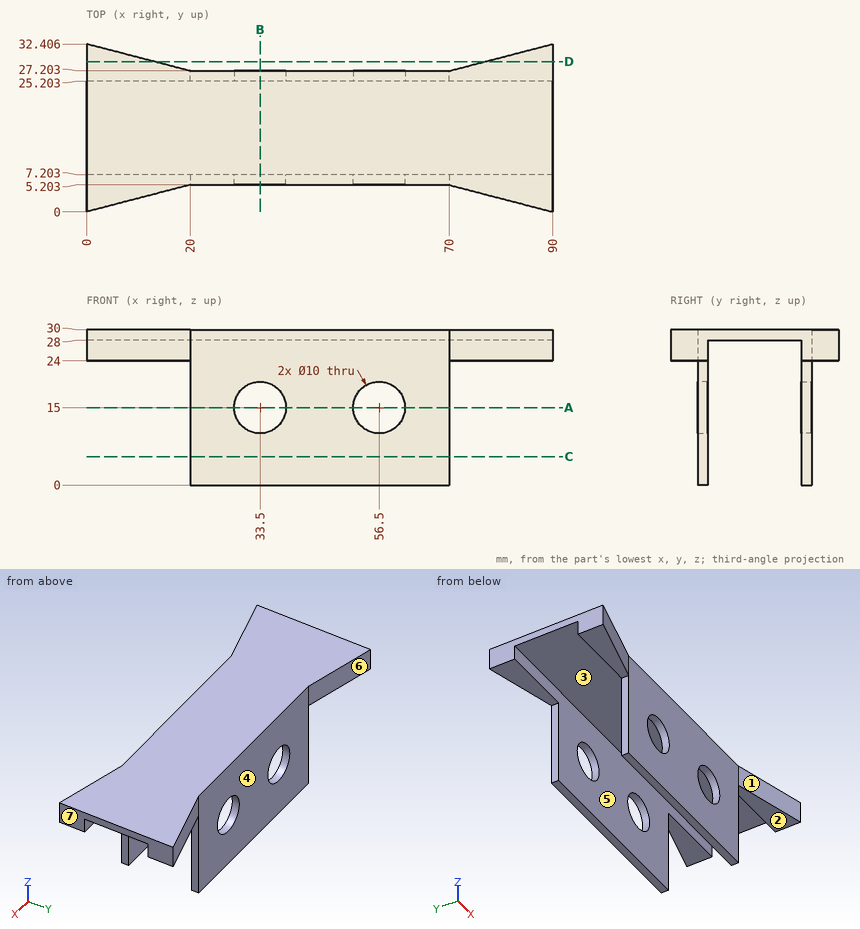
Design review of the part shown in the three views and the two pictorial views. Dimensions are in mm from the part's minimum x, y and z. A direction names the side the tool comes from. Give positions to 0.01 mm unless a question says otherwise; leave off trailing zeros. Write each loop counter-clockwise with the first axis right and the second up, starting at its lowest first coordinate (ties: lowest second). Pieces come first, ordered by that corner, then holes. Notation, with made-up numbers: M 30.5,15.5 L 87.5,15.5 A26 ccw 87.5,40.5 Z; hole C 39.25,72 d11. An arc over 180 degrees is marked long. One line per question, with ' | ' between items. Start each with the question number.
Item 1: For pin 1 (6 mm diameter, centred on x = 78, y = 4.5, fed in from -Z); pin 2 (4 mm diameter, centred on x = 50.5, z = 11, fed in from -Y); pin 3 (1 mm diameter, centred on y = 26, z = 11.5, fed in from +X), all flat-tipped, find the tip position at first contact; note any pin that passes through.
Item 2: Draft analysis for pull direction X (two halves, no side actions). For the marked faces 5, 6 and 7, state which applies: released by +X, released by -X, zero draft, split by the parting line, or undercut.
Item 3: Wall thickness on line 1 (X direction, y = 5.7, z = 15); line 2 (Y direction, x = 50.5, z = 18); line 3 (Z direction, x = 30.5, y = 12): over which ranges is each line inside the solid? List them lowest first. Write a range as from..to.
Item 4: We need section B-B on x = 33.5. Write out the cut boundary in (y, z).
Item 5: For the marked faces 1, 2, 3 and 4, list the 3-axis set-ups (+Z, -Z, +X, -X, +Y, -Y) from which the entire face can be reached by the end or side of a thin tool; tool diameter is ignored.
Item 6: We need section C-C on z = 5.5. Write out the cut boundary in (x, y).
Item 7: We need section A-A on z = 15. Write out the cut boundary in (x, y).
Item 8: We need section D-D on y = 29. Write out the cut boundary in (x, z).
Results found:
1) pin 1: stops at z = 24 | pin 2: stops at y = 5.2 | pin 3: stops at x = 70
2) face 5: zero draft | face 6: undercut | face 7: released by +X
3) line 1: x = 20..28.5, 38.5..51.5, 61.5..70 | line 2: y = 5.2..7.2, 25.2..27.2 | line 3: z = 28..30
4) outline: M 5.2,0 L 7.2,0 L 7.2,10 L 5.2,10 Z; M 5.2,20 L 7.2,20 L 7.2,28 L 25.2,28 L 25.2,20 L 27.2,20 L 27.2,30 L 5.2,30 Z; M 25.2,0 L 27.2,0 L 27.2,10 L 25.2,10 Z
5) face 1: +Z, -Z, -Y | face 2: -Z, +X, +Y, -Y | face 3: -Z, +X, -X | face 4: +Z, -Z, +Y
6) outline: M 20,5.2 L 70,5.2 L 70,7.2 L 20,7.2 Z; M 20,25.2 L 70,25.2 L 70,27.2 L 20,27.2 Z
7) outline: M 20,5.2 L 28.5,5.2 L 28.5,7.2 L 20,7.2 Z; M 20,25.2 L 28.5,25.2 L 28.5,27.2 L 20,27.2 Z; M 38.5,5.2 L 51.5,5.2 L 51.5,7.2 L 38.5,7.2 Z; M 38.5,25.2 L 51.5,25.2 L 51.5,27.2 L 38.5,27.2 Z; M 61.5,5.2 L 70,5.2 L 70,7.2 L 61.5,7.2 Z; M 61.5,25.2 L 70,25.2 L 70,27.2 L 61.5,27.2 Z
8) outline: M 0,24 L 13.09,24 L 13.09,30 L 0,30 Z; M 76.91,24 L 90,24 L 90,30 L 76.91,30 Z
